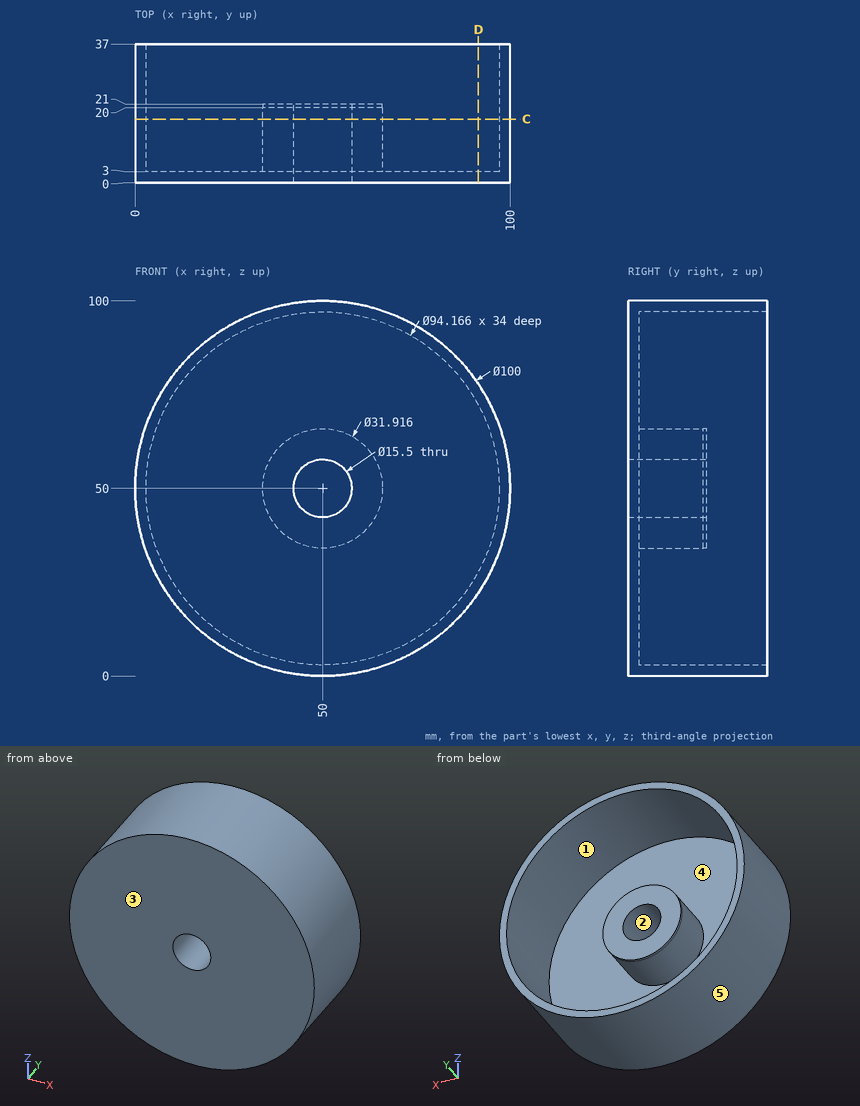
Design review of the part shown in the three views and the two pictorial views. Dimensions are in mm from the part's minimum x, y and z. A direction names the side the tool comes from. Give positions to 0.01 mm unless a question says otherwise; leave off trailing zeros. Loops run counter-clockwise (first coordinate to the right, second up) from the corner with the lowest first, then second, coordinate; pieces in that order, holes last. Notation, with made-up numbers: M 32.25,22 L 83.25,22 A5 cw 83.25,28 Z; hole C -18.5,45.25 d7. An arc over 180 degrees is marked long. Write item = value, one per line.
Q1. To check wall thickness, follow line 1 (X direction, y = 12, z = 50); line 2 (Z direction, x = 49.5, y = 17). State the ranges of each line that lie inside material, in increasing order. Write a range as [from, to].
Output values:
line_1 = [0, 2.92], [34.04, 42.25], [57.75, 65.96], [97.08, 100]
line_2 = [0, 2.92], [34.05, 42.27], [57.73, 65.95], [97.08, 100]
Q2. For the marked faces 1 and 2, list the 3-axis set-ups (+Z, -Z, +X, -X, +Y, -Y) from which the entire face can be reached by the end or side of a thin tool; tool diameter is ignored.
Output values:
face_1 = +Y
face_2 = +Y, -Y
Q3. We need section C-C (y = 17). Count the separate pieces of the cut face and the enclosed holes in it, plus the area to 3 significant figures.
Output values:
separate_pieces = 2
enclosed_holes = 2
area = 1,500 mm^2
Q4. Insertion check: pin 1 (3 mm diameter, centred on x = 88, y = 20.5, fed in from +Z); pin 2 (12 mm diameter, centred on y = 27.5, z = 60.5, fed in from +X); pin 3 (16 mm diameter, centred on x = 46.5, z = 51.5, fed in from +Y). Each pin has a flat end and moves straight along its axis. Give the tip position at first contact, or say it passes through.
Output values:
pin_1 = 84.17
pin_2 = 99.8
pin_3 = 21
Q5. We need section D-D (x = 91.5). Give the boundary of the cut face in (y, z).
Output values:
outline = M 0,22.11 L 37,22.11 L 37,27.76 L 3,27.76 L 3,72.24 L 37,72.24 L 37,77.89 L 0,77.89 Z
Q6. Draft analysis for pull direction Z (two halves, no side actions). For the marked faces 3, 4 and 5, state which applies: +Z half, -Z half, draft (parallel to the pull), parting line (faces both ways), or undercut.
Output values:
face_3 = draft
face_4 = undercut
face_5 = parting line
